Here's how the part is built. I have some questions about the finished solid (model axes, mm). Coordinates: 2 decimals unless noted, no trailing zeros. Write each loop counter-clockwise with the first axis right and the second up, starting at its lowest first coordinate (ties: lowest second). Pieces come first, ordered by that corner, then holes. Notation, with made-up numbers: M 51.5,36 L 65.5,36 A23 cw 65.5,47 Z; hole C 84,6 d4. An arc over 180 degrees is marked long. Use a Markdown table: item, result.
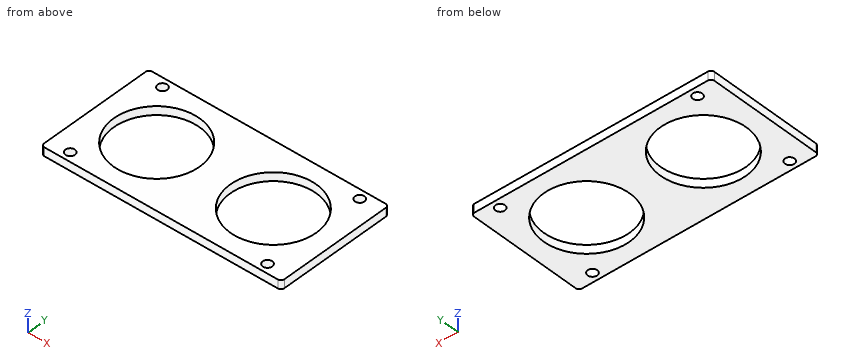
Autodesk Inventor part; units mm, degrees
ref_plane "YZ Plane" through (0, 0, 0) normal (1, 0, 0) x (0, 1, 0)
ref_plane "XZ Plane" through (0, 0, 0) normal (0, 1, 0) x (-1, 0, 0)
ref_plane "XY Plane" through (0, 0, 0) normal (0, 0, 1) x (1, 0, 0)
sketch "Sketch1" plane through (0, 0, 0) normal (0, 0, 1) x (1, 0, 0)
  line L0 (-70, -35) -> (70, -35)
  line L1 (70, -35) -> (70, 35)
  line L2 (70, 35) -> (-70, 35)
  line L3 (-70, 35) -> (-70, -35)
  line L4 (-70, -35) -> (70, 35) construction
  line L5 (70, -35) -> (-70, 35) construction
  point P0 (0, 0)
  dimension "d0" = 140
  dimension "d1" = 70
extrude "Extrusion1" add sketch "Sketch1" along normal blind 5
sketch "Sketch2" plane through (0, 0, 5) normal (0, 0, 1) x (1, 0, 0)
  line L0 (-57.5, -30) -> (57.5, -30) construction
  line L1 (57.5, -30) -> (57.5, 30) construction
  line L2 (57.5, 30) -> (-57.5, 30) construction
  line L3 (-57.5, 30) -> (-57.5, -30) construction
  line L4 (-57.5, -30) -> (57.5, 30) construction
  line L5 (57.5, -30) -> (-57.5, 30) construction
  point P0 (0, 0)
  dimension "d4" = 115
  dimension "d5" = 60
hole "Hole1" at (-57.5, -30, 5) at (-57.5, 30, 5) at (57.5, 30, 5) at (57.5, -30, 5) direction (0, 0, -1) diameter 5.5 depth 8 tip angle 118
fillet "Fillet1" radius 2 4 edges at (70, 35, 2.5) (70, -35, 2.5) (-70, 35, 2.5) (-70, -35, 2.5)
sketch "Sketch3" plane through (0, 0, 5) normal (0, 0, 1) x (1, 0, 0)
  circle A0 centre (-34, 0) radius 25
  circle A1 centre (34, 0) radius 25
  line L0 (-34, 0) -> (34, 0) construction
  point P0 (0, 0)
  point P1 (0, 0)
  dimension "d14" = 50
  dimension "d15" = 50
  dimension "d16" = 68
extrude "Extrusion2" cut sketch "Sketch3" against normal blind 5
properties part number "EndStück_Caps" material "Polycarbonate, Clear"
1. I need wall thicknesses on probe 1 along X at (y, z) = (-30, 2.65); probe 2 along X at (y, z) = (-28, 3.4); probe 3 along Y at (x, z) = (-34, 3.15). Which ranges of each line are inside material? Lowest first, please.
Answers follow:
| item | result |
|---|---|
| probe 1 | x = -70 to -60.25, -54.75 to 54.75, 60.25 to 70 |
| probe 2 | x = -70 to -59.39, -55.61 to 55.61, 59.39 to 70 |
| probe 3 | y = -35 to -25, 25 to 35 |
2. Suppose I cut it at B-B on y = 0. Write out the boundary of the cut face in (x, z), and give its area (3 significant figures).
Answers follow:
| item | result |
|---|---|
| outline | M -70,0 L -59,0 L -59,5 L -70,5 Z; M -9,0 L 9,0 L 9,5 L -9,5 Z; M 59,0 L 70,0 L 70,5 L 59,5 Z |
| area | 200 mm2 |
3. Suppose I cut it at D-D on x = 49. Write out the boundary of the cut face in (y, z).
Answers follow:
| item | result |
|---|---|
| outline | M -35,0 L -20,0 L -20,5 L -35,5 Z; M 20,0 L 35,0 L 35,5 L 20,5 Z |
4. Suppose I cut it at A-A on x = 34. Write out the boundary of the cut face in (y, z), and give its area (3 significant figures).
Answers follow:
| item | result |
|---|---|
| outline | M -35,0 L -25,0 L -25,5 L -35,5 Z; M 25,0 L 35,0 L 35,5 L 25,5 Z |
| area | 100 mm2 |
5. Suppose I cut it at C-C on z = 1.3. Write out the boundary of the cut face in (x, y), and give its area (3 significant figures).
Answers follow:
| item | result |
|---|---|
| outline | M -70,-33 A2 ccw -68,-35 L 68,-35 A2 ccw 70,-33 L 70,33 A2 ccw 68,35 L -68,35 A2 ccw -70,33 Z; hole C -57.5,-30 d5.5; hole C -57.5,30 d5.5; hole C -34,0 d50; hole C 34,0 d50; hole C 57.5,-30 d5.5; hole C 57.5,30 d5.5 |
| area | 5,770 mm2 |
